Geometry: final body of the model. Coordinates: model frame, mm. Face numbers are marked on the shaded views. Round coordinates to 2 decimals unless told otherwise and drop trailing zeros. Loops run counter-clockwise (first coordinate to the right, second up) from the corner with the lowest first, then second, coordinate; pieces in that order, holes last. Notation, with made-up numbers: (61.25, 65) - (68.25, 65) arc R33 ccw to (68.25, 100) - close; hole circle Ø8 at (61.5, 67). An arc over 180 degrees is marked (long way). Use CSV: the item, a comma, the result in double quotes.
from build123d import *

# Parameters (mm, degrees)
F0_R     = 13
F0_R_2   = 7.75
F1_DEPTH = 3.5
F2_SIZE2 = 0.5
F2_SIZE  = 0.5


with BuildPart() as f1:
    # F0 (on Front) → F1 (new body)
    with BuildSketch(Plane.XZ):
        Circle(F0_R)
        Circle(F0_R_2, mode=Mode.SUBTRACT)
    extrude(amount=F1_DEPTH)

    # F2
    f2_edges = [f1.edges().sort_by_distance(p)[0] for p in [
        (-13, -3.5, 0),
        (-7.75, -3.5, 0),
        (-13, 0, 0),
        (-7.75, 0, 0),
    ]]
    chamfer(f2_edges, length=F2_SIZE, length2=F2_SIZE2)


solid = f1.part
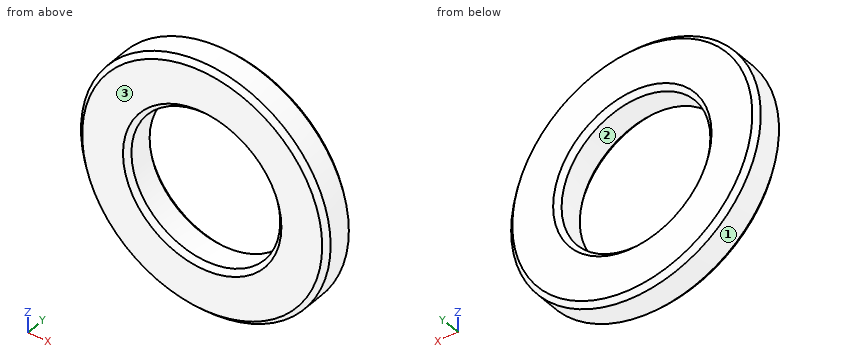
Item 1: Pin query (flat end, axial travel): P1, Ø1.5, axis at y = -2, z = 3.5, coming from the -X side; P2, Ø14, axis at x = 0, z = 0, coming from the +Y side. Return the tip coordinate at first contact, or that it passes through.
Final values:
P1,"stops at x = -12.71"
P2,"passes through"
Item 2: Section B-B on z = 0. Return the cut outline in (x, y).
Final values:
outline,"(-13, -3) - (-12.5, -3.5) - (-8.25, -3.5) - (-7.75, -3) - (-7.75, -0.5) - (-8.25, 0) - (-12.5, 0) - (-13, -0.5) - close; (7.75, -3) - (8.25, -3.5) - (12.5, -3.5) - (13, -3) - (13, -0.5) - (12.5, 0) - (8.25, 0) - (7.75, -0.5) - close"
Item 3: Section A-A on x = 0. Return the cut outline in (y, z), plus the area to 4 significant figures.
Final values:
outline,"(-3.5, -12.5) - (-3, -13) - (-0.5, -13) - (0, -12.5) - (0, -8.25) - (-0.5, -7.75) - (-3, -7.75) - (-3.5, -8.25) - close; (-3.5, 8.25) - (-3, 7.75) - (-0.5, 7.75) - (0, 8.25) - (0, 12.5) - (-0.5, 13) - (-3, 13) - (-3.5, 12.5) - close"
area,"35.75 mm²"
Item 4: Material intervals for line 1 (Z direction, x = 0, y = -1.6); line 2 (X direction, y = -2.25, z = 5.5); line 3 (Z direction, x = 7, y = -0.6), sorted ascending.
Final values:
line 1,"z = -13 to -7.75, 7.75 to 13"
line 2,"x = -11.78 to -5.46, 5.46 to 11.78"
line 3,"z = -10.95 to -3.33, 3.33 to 10.95"
Item 5: Mould query, pull axis X, two halves, no side actions, for the marked faces 1, 2 and 3. Classes: released by +X, released by -X, zero draft, split by the parting line, or undercut.
Final values:
face 1,"split by the parting line"
face 2,"undercut"
face 3,"zero draft"
